Input: part model. Units: mm. Frame: model coordinates. Face numbers are marked on the shaded views. Coordinates: 2 decimals unless noted, no trailing zeros. Order: outer loops, then holes, each group sorted by start corner. A loop starts at its lowest first (then second) coordinate and runs counter-clockwise, first axis right, second up. Notation, with made-up numbers: M 68.25,4.25 L 112.25,4.25 A15 ccw 112.25,16.25 Z; hole C -16,37.25 d2. An arc over 180 degrees is marked long. Answer in a Markdown table with one row per item.
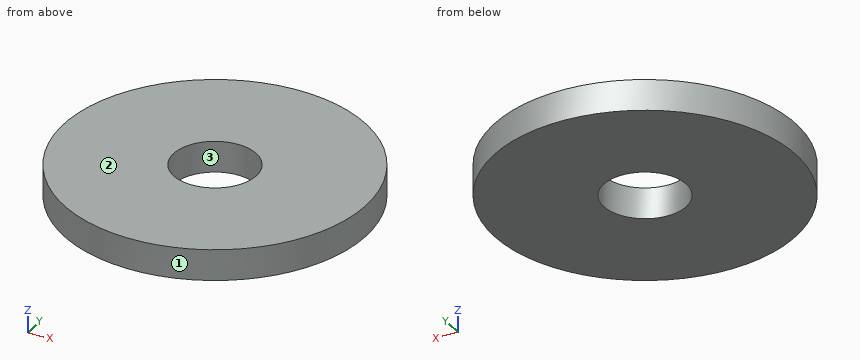
Autodesk Fusion 360 part; units mm, degrees
sketch "Sketch17" plane through (0, 0, 0) normal (0, 0, 1) x (1, 0, 0)
  line L0 (0, 0) -> (0, 10)
  line L1 (0, 10) -> (6, 10)
  line L2 (6, 10) -> (6, 0)
  line L3 (6, 0) -> (0, 0)
  line L4 (0, 8) -> (6, 8)
  line L5 (3, 8) -> (3, 0)
  line L6 (3, 0) -> (3, 3)
  circle A0 centre (3, 3) radius 1
  line L7 (12, 10) -> (12, 0)
  line L8 (9, 0) -> (9, 3)
  line L9 (9, 8) -> (9, 0)
  line L10 (6, 8) -> (12, 8)
  circle A1 centre (9, 3) radius 1
  line L11 (12, 0) -> (6, 0)
  line L12 (6, 0) -> (6, 10)
  line L13 (6, 10) -> (12, 10)
  dimension "d299" = 10
  dimension "d300" = 6
  dimension "d301" = 3
  dimension "d302" = 2
  dimension "d308" = 10
  dimension "d309" = 6
  dimension "d310" = 3
  dimension "d311" = 2
  dimension "d333" = 6
sketch "Sketch18" plane through (0, 0, 0) normal (0, 0, 1) x (1, 0, 0)
  circle A0 centre (6, -8.1962) radius 11.5911
  circle A1 centre (6, -8.1962) radius 13.5911
  circle A2 centre (6, -8.1962) radius 9.5911
  line L0 (6, -8.1962) -> (-5.3131, -0.664)
  circle A3 centre (6, -8.1962) radius 14.5911
  line L1 (6, -8.1962) -> (-6.1795, -14.2275)
  circle A4 centre (6, -8.1962) radius 4
  point P0 (3, 3)
  point P1 (9, 3)
  point P2 (3, 3)
  point P3 (3, 3)
  point P4 (9, 3)
  point P5 (3, 3)
  dimension "d337" = 23.1822
  dimension "d339" = 11.5911
  dimension "d340" = 11.5911
  dimension "d341" = 27.1822
  dimension "d342" = 19.1822
  dimension "d347" = 29.1822
  dimension "d351" = 60
  dimension "d352" = 8
extrude "Extrude45" add sketch "Sketch18" along normal blind 3 contours A0 A2 L0 L1 | A0 A1 L0 L1 picked at (16.8462, -9.2442) picked at (-2.4639, -17.9204) makes body 1
pattern_circular "C-Pattern13" count 3 over 360 about axis through (6, -8.1962, 0) along (0, 0, 1) of bodies 1 makes body 2 at (4.5479, -20.3354, 3) makes body 3 at (6.1044, 4.0292, 0)
extrude "Extrude46" add sketch "Sketch18" along normal blind 3 contours A2 L0 L1 A4 | A2 L0 L1 A4 | A3 bodies 1 2 3
equation "d333 = Linear Dimension-8"
equation "d337 = Diameter Dimension-2"
equation "d339 = Linear Dimension-3"
equation "d340 = Linear Dimension-3"
equation "d341 = Diameter Dimension-3"
equation "d342 = Diameter Dimension-4"
equation "d347 = Diameter Dimension-5"
equation "d351 = C-Pattern1-Angle"
equation "d352 = Diameter Dimension-6"
1) Cut plane D-D, the plane y = 0.5. Output: boundary loops of the cut face in (x, z), and give its area (3 significant figures).
Resolved:
| item | result |
|---|---|
| outline | M -5.72,0 L 17.72,0 L 17.72,3 L -5.72,3 Z |
| area | 70.3 mm2 |
2) Cut plane C-C, the plane z = 1.9. Output: boundary loops of the cut face in (x, y), and give its area (3 significant figures).
Resolved:
| item | result |
|---|---|
| outline | C 6,-8.2 d29.18; hole C 6,-8.2 d8 |
| area | 619 mm2 |
3) Mould query, pull axis Y, two halves, no side actions, for the marked faces 1, 2 and 3. Classes: +Y half, -Y half, draft (parallel to the pull), parting line (faces both ways), or undercut.
Resolved:
| item | result |
|---|---|
| face 1 | parting line |
| face 2 | draft |
| face 3 | undercut |
4) Cut plane A-A, the plane x = 6. Output: boundary loops of the cut face in (y, z).
Resolved:
| item | result |
|---|---|
| outline | M -22.79,0 L -12.2,0 L -12.2,3 L -22.79,3 Z; M -4.2,0 L 6.39,0 L 6.39,3 L -4.2,3 Z |
5) Contact query for flat-ended pins moving along their axis: pin 1 (1.5 mm diameter, centred on x = -2.5, z = 1, fed in from -Y); pin 2 (1 mm diameter, centred on y = -11.5, z = 2.5, fed in from +X); pin 3 (5 mm diameter, centred on x = 6, y = -8.2, fed in from -Z). Output: stop coordinate, or through.
Resolved:
| item | result |
|---|---|
| pin 1 | stops at y = -20.56 |
| pin 2 | stops at x = 20.32 |
| pin 3 | passes through |
6) Material intervals for probe 1 along Y at (x, z) = (6, 0.8); probe 2 along X at (y, z) = (-8.5, 1.55); probe 3 along X at (y, z) = (-6.75, 2.3), sorted ascending.
Resolved:
| item | result |
|---|---|
| probe 1 | y = -22.79 to -12.2, -4.2 to 6.39 |
| probe 2 | x = -8.59 to 2.01, 9.99 to 20.59 |
| probe 3 | x = -8.52 to 2.27, 9.73 to 20.52 |
7) Cut plane B-B, the plane y = -5.5. Output: boundary loops of the cut face in (x, z).
Resolved:
| item | result |
|---|---|
| outline | M -8.34,0 L 3.05,0 L 3.05,3 L -8.34,3 Z; M 8.95,0 L 20.34,0 L 20.34,3 L 8.95,3 Z |
